Autodesk Inventor part; units mm, degrees
ref_plane "h1_XY" through (23.8125, 0, 25.4) normal (1, 0, 0) x (0, 0, -1)
ref_plane "h1_YZ" through (23.8125, 0, 25.4) normal (0, 0, -1) x (0, 1, 0)
ref_plane "h1_ZX" through (23.8125, 0, 25.4) normal (0, 1, 0) x (1, 0, 0)
sketch "Sketch_1" plane through (0, 0, 0) normal (1, 0, 0) x (0, 1, 0)
  line L0 (0, 25.4) -> (0, 4.6228)
  arc A0 (0, 4.6228) -> (4.6228, 0) centre (4.6228, 4.6228) ccw
  line L1 (4.6228, 0) -> (42.0624, 0)
  line L2 (42.0624, 0) -> (42.0624, 3.048)
  line L3 (42.0624, 3.048) -> (4.6228, 3.048)
  arc A1 (3.048, 4.6228) -> (4.6228, 3.048) centre (4.6228, 4.6228) ccw
  line L4 (3.048, 4.6228) -> (3.048, 25.4)
  line L5 (3.048, 25.4) -> (0, 25.4)
extrude "Extrusion1" add sketch "Sketch_1" along normal blind 47.625
sketch "Sketch_2" plane through (0, 0, 0) normal (0, 0, 1) x (1, 0, 0)
  line L0 (-9.525, -3.5052) -> (57.15, -3.5052)
  line L1 (57.15, -3.5052) -> (57.15, 56.0832)
  line L2 (57.15, 56.0832) -> (-9.525, 56.0832)
  line L3 (-9.525, 56.0832) -> (-9.525, -3.5052)
  line L4 (-3.3686, 0) -> (50.9936, 0)
  line L5 (50.9936, 0) -> (36.4228, 27.4668)
  arc A0 (36.4228, 27.4668) -> (11.2022, 27.4668) centre (23.8125, 20.7772) ccw
  line L6 (11.2022, 27.4668) -> (-3.3686, 0)
extrude "Extrusion2" cut sketch "Sketch_2" along normal blind 4.572
sketch "Sketch_3" plane through (0, 0, 0) normal (0, 0, 1) x (1, 0, 0)
  circle A0 centre (23.8125, 20.574) radius 7.9883
extrude "Extrusion3" cut sketch "Sketch_3" along normal blind 4.572
sketch "Sketch_6" plane through (0, 0, 0) normal (0, 1, 0) x (-1, 0, 0)
  line L0 (23.8125, 22.225) -> (23.8125, 32.512)
  line L1 (23.8125, 32.512) -> (-3.175, 32.512)
  line L2 (-3.175, 32.512) -> (-3.175, 25.4)
  arc A0 (0, 22.225) -> (-3.175, 25.4) centre (-3.175, 22.225) ccw
  line L3 (0, 22.225) -> (23.8125, 22.225)
extrude "Extrusion4" cut sketch "Sketch_6" along normal blind 4.572
sketch "Sketch_7" plane through (0, 0, 0) normal (0, 1, 0) x (-1, 0, 0)
  line L0 (-44.45, 32.512) -> (-71.4375, 32.512)
  line L1 (-71.4375, 32.512) -> (-71.4375, 22.225)
  line L2 (-71.4375, 22.225) -> (-47.625, 22.225)
  arc A0 (-44.45, 25.4) -> (-47.625, 22.225) centre (-44.45, 22.225) ccw
  line L3 (-44.45, 25.4) -> (-44.45, 32.512)
extrude "Extrusion5" cut sketch "Sketch_7" along normal blind 4.572
sketch "Sketch_8" plane through (0, 0, 0) normal (0, 1, 0) x (-1, 0, 0)
  line L0 (4.7625, 17.6022) -> (-4.7625, 17.6022)
  arc A0 (-4.7625, 17.6022) -> (-4.7625, 10.8458) centre (-4.7625, 14.224) ccw
  line L1 (-4.7625, 10.8458) -> (4.7625, 10.8458)
  line L2 (4.7625, 10.8458) -> (4.7625, 17.6022)
extrude "Extrusion6" cut sketch "Sketch_8" along normal blind 4.572
sketch "Sketch_9" plane through (0, 0, 0) normal (0, 1, 0) x (-1, 0, 0)
  arc A0 (-42.8625, 10.8458) -> (-42.8625, 17.6022) centre (-42.8625, 14.224) ccw
  line L0 (-42.8625, 17.6022) -> (-52.3875, 17.6022)
  line L1 (-52.3875, 17.6022) -> (-52.3875, 10.8458)
  line L2 (-52.3875, 10.8458) -> (-42.8625, 10.8458)
extrude "Extrusion7" cut sketch "Sketch_9" along normal blind 4.572
ref_plane "h1_XY" through (23.8125, 0, 25.4) normal (1, 0, 0) x (0, 0, -1)
ref_plane "h1_YZ" through (23.8125, 0, 25.4) normal (0, 0, -1) x (0, 1, 0)
ref_plane "h1_ZX" through (23.8125, 0, 25.4) normal (0, 1, 0) x (1, 0, 0)
ref_plane "d1_XY" through (23.8125, 12.5857, 0) normal (1, 0, 0) x (0, 0, -1)
ref_plane "d1_YZ" through (23.8125, 12.5857, 0) normal (0, 0, -1) x (0, 1, 0)
ref_plane "d1_ZX" through (23.8125, 12.5857, 0) normal (0, 1, 0) x (1, 0, 0)
ref_plane "h2_XY" through (23.8125, 3.048, 25.4) normal (1, 0, 0) x (0, 0, -1)
ref_plane "h2_YZ" through (23.8125, 3.048, 25.4) normal (0, 0, -1) x (0, 1, 0)
ref_plane "h2_ZX" through (23.8125, 3.048, 25.4) normal (0, 1, 0) x (1, 0, 0)
ref_plane "d2_XY" through (23.8125, 28.5623, 0) normal (1, 0, 0) x (0, 0, -1)
ref_plane "d2_YZ" through (23.8125, 28.5623, 0) normal (0, 0, -1) x (0, 1, 0)
ref_plane "d2_ZX" through (23.8125, 28.5623, 0) normal (0, 1, 0) x (1, 0, 0)
ref_plane "h3_XY" through (23.8125, 20.574, 3.048) normal (1, 0, 0) x (0, 0, -1)
ref_plane "h3_YZ" through (23.8125, 20.574, 3.048) normal (0, 0, -1) x (0, 1, 0)
ref_plane "h3_ZX" through (23.8125, 20.574, 3.048) normal (0, 1, 0) x (1, 0, 0)
ref_plane "h4_XY" through (23.8125, 35.052, 3.048) normal (1, 0, 0) x (0, 0, -1)
ref_plane "h4_YZ" through (23.8125, 35.052, 3.048) normal (0, 0, -1) x (0, 1, 0)
ref_plane "h4_ZX" through (23.8125, 35.052, 3.048) normal (0, 1, 0) x (1, 0, 0)
ref_plane "h5_XY" through (47.625, 6.35, 0) normal (1, 0, 0) x (0, 0, -1)
ref_plane "h5_YZ" through (47.625, 6.35, 0) normal (0, 0, -1) x (0, 1, 0)
ref_plane "h5_ZX" through (47.625, 6.35, 0) normal (0, 1, 0) x (1, 0, 0)
ref_plane "h6_XY" through (47.625, 0, 0) normal (1, 0, 0) x (0, 0, -1)
ref_plane "h6_YZ" through (47.625, 0, 0) normal (0, 0, -1) x (0, 1, 0)
ref_plane "h6_ZX" through (47.625, 0, 0) normal (0, 1, 0) x (1, 0, 0)
ref_plane "l1_XY" through (0, 0, 0) normal (0, 1, 0) x (1, 0, 0)
ref_plane "l1_YZ" through (0, 0, 0) normal (1, 0, 0) x (0, 0, -1)
ref_plane "l1_ZX" through (0, 0, 0) normal (0, 0, -1) x (0, 1, 0)
ref_plane "l2_XY" through (47.625, 0, 0) normal (0, 1, 0) x (1, 0, 0)
ref_plane "l2_YZ" through (47.625, 0, 0) normal (1, 0, 0) x (0, 0, -1)
ref_plane "l2_ZX" through (47.625, 0, 0) normal (0, 0, -1) x (0, 1, 0)
ref_plane "l3_XY" through (0, 0, 25.4) normal (0, 1, 0) x (1, 0, 0)
ref_plane "l3_YZ" through (0, 0, 25.4) normal (1, 0, 0) x (0, 0, -1)
ref_plane "l3_ZX" through (0, 0, 25.4) normal (0, 0, -1) x (0, 1, 0)
ref_plane "l4_XY" through (0, 0, 14.224) normal (0, 1, 0) x (1, 0, 0)
ref_plane "l4_YZ" through (0, 0, 14.224) normal (1, 0, 0) x (0, 0, -1)
ref_plane "l4_ZX" through (0, 0, 14.224) normal (0, 0, -1) x (0, 1, 0)
ref_plane "l5_XY" through (4.7625, 0, 14.224) normal (0, 1, 0) x (1, 0, 0)
ref_plane "l5_YZ" through (4.7625, 0, 14.224) normal (1, 0, 0) x (0, 0, -1)
ref_plane "l5_ZX" through (4.7625, 0, 14.224) normal (0, 0, -1) x (0, 1, 0)
ref_plane "l6_XY" through (42.8625, 0, 14.224) normal (0, 1, 0) x (1, 0, 0)
ref_plane "l6_YZ" through (42.8625, 0, 14.224) normal (1, 0, 0) x (0, 0, -1)
ref_plane "l6_ZX" through (42.8625, 0, 14.224) normal (0, 0, -1) x (0, 1, 0)
ref_plane "l7_XY" through (42.8625, 0, 17.6022) normal (0, 1, 0) x (1, 0, 0)
ref_plane "l7_YZ" through (42.8625, 0, 17.6022) normal (1, 0, 0) x (0, 0, -1)
ref_plane "l7_ZX" through (42.8625, 0, 17.6022) normal (0, 0, -1) x (0, 1, 0)
ref_plane "l8_XY" through (42.8625, 0, 10.8458) normal (0, 1, 0) x (1, 0, 0)
ref_plane "l8_YZ" through (42.8625, 0, 10.8458) normal (1, 0, 0) x (0, 0, -1)
ref_plane "l8_ZX" through (42.8625, 0, 10.8458) normal (0, 0, -1) x (0, 1, 0)
ref_plane "mounting_bracket_XY" through (23.8125, 20.574, 3.048) normal (0, 0, 1) x (1, 0, 0)
ref_plane "mounting_bracket_YZ" through (23.8125, 20.574, 3.048) normal (1, 0, 0) x (0, 1, 0)
ref_plane "mounting_bracket_ZX" through (23.8125, 20.574, 3.048) normal (0, 1, 0) x (0, 0, 1)
ref_plane "mounting_bracket_1_XY" through (23.8125, 20.574, 0) normal (0, 0, 1) x (1, 0, 0)
ref_plane "mounting_bracket_1_YZ" through (23.8125, 20.574, 0) normal (1, 0, 0) x (0, 1, 0)
ref_plane "mounting_bracket_1_ZX" through (23.8125, 20.574, 0) normal (0, 1, 0) x (0, 0, 1)
properties part number "D-129"
Build history of the part. All positions in model axes, mm. A direction names the side the tool comes from. Round coordinates to 2 decimals unless told otherwise and drop trailing zeros. Write each loop counter-clockwise with the first axis right and the second up, starting at its lowest first coordinate (ties: lowest second). Pieces come first, ordered by that corner, then holes. Notation, with made-up numbers: M 52,24 L 103,24 A20 cw 103,38 Z; hole C -35.5,30.25 d7. An arc over 180 degrees is marked long. Answer as a JSON object with one key per item and string values. Group by question number.
(1) Cut at C-C (x = 38). Give the cut face in (y, z), and give its area (3 significant figures).
(2) Mould opens along Z. For faces 1 (the flat face through (29, 13, 3.048)), 2 (the cylindrical face through (31.43, 18.17, 1.5)), 3 (the flat face through (2, 2, 10.846)) say: pulls with the +Z half, pulls with the -Z half, needs draft (parallel to the pull), parting line crosses it, or undercut.
(3) Drill centre line: L1, parallel to Z at x = 24.5, y = 5.5. Where is it in solid material? Low to high.
(4) Flat gauge pins, fed straight in: pin 1 (10.5 mm diameter, centred on x = 18, z = 15.5, fed in from +Y); pin 2 (4 mm diameter, centred on y = 6.5, z = 6.5, fed in from -X); pin 3 (0.9 mm diameter, centred on x = 45, y = 1.5, fed in from -Z); pin 4 (4 mm diameter, centred on x = 16, y = 5.5, fed in from +Z). Where does each tip first touch, or does it go through?
(5) Cut at B-B (y = 18). Give the cut face in (x, z), and give its area (3 significant figures).
(6) Which spindle directions (+Z, -Z, +X, -X, +Y, -Y) get a long thin tool onto all of the face, cutting with end or side? Do faces 4 (the flat face through (0, 2, 4)), 5 (the flat face through (45, 2, 10.846)), 6 (the flat face through (47.625, 2, 4)), 7 (the flat face through (2, 2, 17.602)), 8 (the flat face through (23, 3.048, 15)). Say none if no direction does.
(7) Cut at A-A (x = 30.5). Give the cut face in (y, z), and give its area (3 significant figures).
Responses:
{
 "1": {"outline": "M 0,4.62 A4.62 ccw 4.62,0 L 24.49,0 L 24.49,3.05 L 4.62,3.05 A1.57 cw 3.05,4.62 L 3.05,25.4 L 0,25.4 Z", "area": "139 mm2"},
 "2": {"face 1": "pulls with the +Z half", "face 2": "needs draft", "face 3": "undercut"},
 "3": {"L1": "z = 0 to 3.05"},
 "4": {"pin 1": "stops at y = 3.05", "pin 2": "passes through", "pin 3": "stops at z = 0.85", "pin 4": "stops at z = 3.52"},
 "5": {"outline": "M 6.18,0 L 16.25,0 L 16.25,3.05 L 6.18,3.05 Z; M 31.37,0 L 41.44,0 L 41.44,3.05 L 31.37,3.05 Z", "area": "61.4 mm2"},
 "6": {"face 4": "+Z, -Z, -X, +Y, -Y", "face 5": "+X, +Y, -Y", "face 6": "+Z, -Z, +X, +Y, -Y", "face 7": "-X, +Y, -Y", "face 8": "+Z, +X, -X, +Y"},
 "7": {"outline": "M 0,4.62 A4.62 ccw 4.62,0 L 16.2,0 L 16.2,3.05 L 4.62,3.05 A1.57 cw 3.05,4.62 L 3.05,25.4 L 0,25.4 Z; M 24.94,0 L 33.39,0 L 33.39,3.05 L 24.94,3.05 Z", "area": "139 mm2"}
}
